For this review, take the finished solid that the model builds, in its own axes (mm). A direction names the side the tool comes from. Give positions to 0.01 mm unless a question says otherwise; leave off trailing zeros. Order: outer loops, then holes, each group sorted by start corner. A loop starts at its lowest first (then second) coordinate and runs counter-clockwise, first axis right, second up. Notation, with made-up numbers: (30, 84.25) -> (39, 84.25) arc R11 ccw to (39, 105.25) -> close; hole circle Ø4 at (-6.75, -16). An arc over 180 degrees is marked (long way). One line per item, written item: value. Start each with the question number.
from build123d import *

# Parameters (mm, degrees)
EXTRUDE_1_DEPTH          = 2
SKETCH_17_W              = 31.8
SKETCH_17_H              = 18
CUT_EXTRUDE_1_DEPTH      = 10
CHAMFER_1_SIZE           = 0.5
CHAMFER_3_SIZE           = 0.5
SKETCH_25_W              = 23.840125732
SKETCH_25_H              = 2
CUT_EXTRUDE_5_DEPTH      = 0.4
CUT_EXTRUDE_6_DEPTH      = 6
CUT_EXTRUDE_6_DEPTH_BACK = 6
SKETCH_28_R              = 0.9
EXTRUDE_3_DEPTH          = 1.2
CHAMFER_6_SIZE           = 0.4
SKETCH_29_R              = 1.6
CUT_EXTRUDE_7_DEPTH      = 3.2
SKETCH_30_R              = 3.5
CUT_EXTRUDE_8_DEPTH      = 10
CHAMFER_9_SIZE           = 0.4
FILLET_1_R               = 1
SKETCH_31_R              = 2.55
CUT_EXTRUDE_9_DEPTH      = 2
CHAMFER_10_SIZE          = 0.4
SKETCH_32_R              = 3.5
SKETCH_32_R_2            = 1.6
SKETCH_32_W              = 32.6
SKETCH_32_H              = 29.3
EXTRUDE_5_DEPTH          = 1.4


with BuildPart() as part:
    # Эскиз1 → Бобышка-Вытянуть1 (new body)
    with BuildSketch(Plane.XY):
        Polygon((42.994929839, 15.7), (0.265604814, 15.7), (-0.805070161, 15.7), (-0.805070161, -3.225667373), (-0.805070161, -27.24226554), (-0.805070161, -29), (41.213218599, -29), (42.994929839, -29), (42.994929839, 0), align=None)
    extrude(amount=EXTRUDE_1_DEPTH)

    # Эскиз17 → Вырез-Вытянуть1 (cut)
    with BuildSketch(Plane(origin=(0, 0, 0), x_dir=(-1, 0, 0), z_dir=(0, 0, -1))):
        with Locations((-21.094929839, 0)):
            Rectangle(SKETCH_17_W, SKETCH_17_H)
    extrude(amount=-CUT_EXTRUDE_1_DEPTH, mode=Mode.SUBTRACT)

    # Фаска1
    chamfer_1_edges = [part.edges().sort_by_distance(p)[0] for p in [
        (36.994929839, 0, 0),
        (21.094929839, -9, 0),
        (5.194929839, 0, 0),
        (21.094929839, 9, 0),
    ]]
    chamfer(chamfer_1_edges, length=CHAMFER_1_SIZE)

    # Фаска3
    chamfer_3_edges = [part.edges().sort_by_distance(p)[0] for p in [
        (21.094929839, 15.7, 0),
        (42.994929839, -6.65, 0),
        (21.094929839, -29, 0),
        (-0.805070161, -6.65, 0),
    ]]
    chamfer(chamfer_3_edges, length=CHAMFER_3_SIZE)

    # Эскиз25 → Вырез-Вытянуть5 (cut)
    with BuildSketch(Plane.XY.offset(2)):
        with Locations((22.524068439, -12.5)):
            Rectangle(SKETCH_25_W, SKETCH_25_H)
    extrude(amount=-CUT_EXTRUDE_5_DEPTH, mode=Mode.SUBTRACT)

    # Эскиз27 → Вырез-Вытянуть6 (cut, two sides: drawn at the far end of the back side and taken through both)
    with BuildSketch(Plane(origin=(0, 0.1, 0), x_dir=(-1, 0, 0), z_dir=(0, -1, 0)).offset(-CUT_EXTRUDE_6_DEPTH_BACK)):
        Polygon((-36.994929839, -2), (-36.994929839, -1.2), (-37.794929839, -2), align=None)
    extrude(amount=CUT_EXTRUDE_6_DEPTH + CUT_EXTRUDE_6_DEPTH_BACK, mode=Mode.SUBTRACT)

    # Эскиз28 → Бобышка-Вытянуть3 (add)
    with BuildSketch(Plane.XY.offset(2)):
        with Locations((7.894929839, 11.5)):
            Circle(SKETCH_28_R)
        with Locations((34.294929839, 11.5)):
            Circle(SKETCH_28_R)
        with Locations(Location((34.294929839, -11.5, 0), (0, 0, 180))):
            Circle(SKETCH_28_R)
        with Locations((7.894929839, -11.5)):
            Circle(SKETCH_28_R)
    extrude(amount=EXTRUDE_3_DEPTH)

    # Фаска6
    chamfer_6_edges = [part.edges().sort_by_distance(p)[0] for p in [
        (21.094929839, 9, 2),
        (21.094929839, -9, 2),
    ]]
    chamfer(chamfer_6_edges, length=CHAMFER_6_SIZE)

    # Эскиз29 → Вырез-Вытянуть7 (cut)
    with BuildSketch(Plane.XY.offset(2)):
        with Locations((2.594929839, 12.3)):
            Circle(SKETCH_29_R)
        with Locations((39.594929839, 12.3)):
            Circle(SKETCH_29_R)
        with Locations((39.594929839, -25.6)):
            Circle(SKETCH_29_R)
    extrude(amount=-CUT_EXTRUDE_7_DEPTH, mode=Mode.SUBTRACT)

    # Эскиз30 → Вырез-Вытянуть8 (cut)
    with BuildSketch(Plane.XY.offset(2)):
        with Locations((8.194929839, -21)):
            Circle(SKETCH_30_R)
    extrude(amount=-CUT_EXTRUDE_8_DEPTH, mode=Mode.SUBTRACT)

    # Фаска9
    chamfer_9_edges = [part.edges().sort_by_distance(p)[0] for p in [
        (4.694929839, -21, 0),
    ]]
    chamfer(chamfer_9_edges, length=CHAMFER_9_SIZE)

    # Скругление1
    # the kernel refuses this fillet: 1 mm, written as the material it takes off along each edge
    with BuildSketch(Plane(origin=(42.994929839, -29, -2), x_dir=(0, 1, 0), z_dir=(0, 0, 1)), Plane(origin=(42.994929839, 15.7, -2), x_dir=(-1, 0, 0), z_dir=(0, 0, 1))) as fillet_1_piece_1:
        with BuildLine():
            CenterArc((FILLET_1_R, FILLET_1_R), FILLET_1_R, 180, 90)
            Line((0, FILLET_1_R), (0, 0))
            Line((0, 0), (FILLET_1_R, 0))
        make_face()
    extrude(amount=6.5, mode=Mode.SUBTRACT)
    with BuildSketch(Plane(origin=(-0.805070161, -29, -2), x_dir=(0, 1, 0), z_dir=(0, 0, 1)), Plane(origin=(-0.805070161, 15.7, -2), x_dir=(1, 0, 0), z_dir=(0, 0, 1))) as fillet_1_piece_2:
        with BuildLine():
            CenterArc((FILLET_1_R, -FILLET_1_R), FILLET_1_R, 90, 90)
            Line((0, -FILLET_1_R), (0, 0))
            Line((0, 0), (FILLET_1_R, 0))
        make_face()
    extrude(amount=6.5, mode=Mode.SUBTRACT)
    with BuildSketch(Plane(origin=(0.528263172, 14.366666667, -0.833333333), x_dir=(0.816496580927726, 0.4082482904638629, 0.4082482904638631), z_dir=(-0.5773502691896258, 0.5773502691896258, 0.5773502691896258)), Plane(origin=(0.528263172, -27.666666667, -0.833333333), x_dir=(-0.4082482904638631, 0.8164965809277261, 0.4082482904638631), z_dir=(-0.5773502691896258, -0.5773502691896258, 0.5773502691896258))) as fillet_1_piece_3:
        with BuildLine():
            CenterArc((FILLET_1_R * 0.57735026919, -FILLET_1_R), FILLET_1_R, 90, 60)
            Line((-FILLET_1_R * 0.288675134595, -FILLET_1_R * 0.5), (0, 0))
            Line((0, 0), (FILLET_1_R * 0.57735026919, 0))
        make_face()
    extrude(amount=3.75277675, mode=Mode.SUBTRACT)
    with BuildSketch(Plane(origin=(41.661596505, 14.366666667, -0.833333333), x_dir=(-0.8164965809277261, 0.4082482904638622, 0.4082482904638635), z_dir=(0.5773502691896256, 0.577350269189626, 0.577350269189626)), Plane(origin=(41.661596505, -27.666666667, -0.833333333), x_dir=(0.4082482904638636, 0.8164965809277261, 0.40824829046386224), z_dir=(0.5773502691896261, -0.5773502691896256, 0.5773502691896256))) as fillet_1_piece_4:
        with BuildLine():
            CenterArc((FILLET_1_R * 0.57735026919, FILLET_1_R), FILLET_1_R, 210, 60)
            Line((-FILLET_1_R * 0.288675134595, FILLET_1_R * 0.5), (0, 0))
            Line((0, 0), (FILLET_1_R * 0.57735026919, 0))
        make_face()
    extrude(amount=3.75277675, mode=Mode.SUBTRACT)

    # Эскиз31 → Вырез-Вытянуть9 (cut)
    with BuildSketch(Plane(origin=(0, 0, 0), x_dir=(-1, 0, 0), z_dir=(0, 0, -1))):
        with Locations((-39.594929839, 12.3)):
            Circle(SKETCH_31_R)
        with Locations((-2.594929839, 12.3)):
            Circle(SKETCH_31_R)
        with Locations((-39.594929839, -25.6)):
            Circle(SKETCH_31_R)
    extrude(amount=-CUT_EXTRUDE_9_DEPTH, mode=Mode.SUBTRACT)

    # Фаска10
    # the kernel refuses this chamfer: 0.4 mm, written as the material it takes off along each edge
    with BuildSketch(Plane(origin=(39.594929839, -25.6, 0), x_dir=(-1, 0, 0), z_dir=(0, -1, 0))) as chamfer_10_piece_1:
        Polygon((2.55 + CHAMFER_10_SIZE, 0), (2.55, -CHAMFER_10_SIZE), (2.55, 0), align=None)
    revolve(axis=Axis((39.594929839, -25.6, 0), (0, 0, -1)), mode=Mode.SUBTRACT)
    with BuildSketch(Plane(origin=(2.594929839, 12.3, 0), x_dir=(-1, 0, 0), z_dir=(0, -1, 0))) as chamfer_10_piece_2:
        Polygon((2.55 + CHAMFER_10_SIZE, 0), (2.55, -CHAMFER_10_SIZE), (2.55, 0), align=None)
    revolve(axis=Axis((2.594929839, 12.3, 0), (0, 0, -1)), mode=Mode.SUBTRACT)
    with BuildSketch(Plane(origin=(39.594929839, 12.3, 0), x_dir=(-1, 0, 0), z_dir=(0, -1, 0))) as chamfer_10_piece_3:
        Polygon((2.55 + CHAMFER_10_SIZE, 0), (2.55, -CHAMFER_10_SIZE), (2.55, 0), align=None)
    revolve(axis=Axis((39.594929839, 12.3, 0), (0, 0, -1)), mode=Mode.SUBTRACT)

    # Эскиз32 → Бобышка-Вытянуть5 (add)
    with BuildSketch(Plane.XY.offset(2)):
        with BuildLine():
            Line((-0.805070161, 14.7), (-0.805070161, -28))
            ThreePointArc((-0.805070161, -28), (-0.512176942, -28.707106781), (0.194929839, -29))
            Line((0.194929839, -29), (41.994929839, -29))
            ThreePointArc((41.994929839, -29), (42.70203662, -28.707106781), (42.994929839, -28))
            Line((42.994929839, -28), (42.994929839, 14.7))
            ThreePointArc((42.994929839, 14.7), (42.70203662, 15.407106781), (41.994929839, 15.7))
            Line((41.994929839, 15.7), (0.194929839, 15.7))
            ThreePointArc((0.194929839, 15.7), (-0.512176942, 15.407106781), (-0.805070161, 14.7))
        make_face()
        with Locations((8.194929839, -21)):
            Circle(SKETCH_32_R, mode=Mode.SUBTRACT)
        with Locations((39.594929839, -25.6)):
            Circle(SKETCH_32_R_2, mode=Mode.SUBTRACT)
        with Locations((39.594929839, 12.3)):
            Circle(SKETCH_32_R_2, mode=Mode.SUBTRACT)
        with Locations((2.594929839, 12.3)):
            Circle(SKETCH_32_R_2, mode=Mode.SUBTRACT)
        with Locations((21.494929839, -0.35)):
            Rectangle(SKETCH_32_W, SKETCH_32_H, mode=Mode.SUBTRACT)
    extrude(amount=EXTRUDE_5_DEPTH)


solid = part.part
Q1. For line 1 along Y through (x, z) = (22, 0.7); line 2 along X through (y, z) = (-3.5, 0.6); line 3 along Y through (x, z) = (16.5, 2.5), list the stretches that pass through material, from the lowest coordinate up.
Q2. For pin 1 Ø5.5 at (x, y) = (8.19, -21) entering from +Z; pin 2 Ø1.4 at (x, y) = (8, -11.5) entering from +Z; pin 3 Ø4.5 at (x, y) = (14.5, -10.5) entering from +Z, all flat-tipped, find the tip position at first contact; note any pin that passes through.
Q3. Take a section at A-A (x = 19.5). State the section outline as (y, z) points.
Q4. Take a section at B-B (y = -21). State the section outline as (x, z) points.
Q5. Mouldability with a two-part tool opening along Y and no side actions: class faces 1 (the flat face through (0, 14, 0)), 2 (the cylindrical face through (7.232, 12.108, 2.592)), 3 (the cylindrical face through (-0.52, -28.7, 1.88)), 4 (the cylindrical face through (38.325, -26.574, 2.69)) as pulls with the +Y half, pulls with the -Y half, needs draft (parallel to the pull), parting line crosses it, or undercut.
Q6. Take a section at D-D (x = 7.5). State how many separate pieces and enclosed holes the cut face has, and give its area (3 significant figures).
Q7. Take a section at C-C (y = -25.6). State the section outline as (x, z) points (3 decimals), and give its area (3 significant figures).
Q8. For faces 5 (the flat face through (21, -15, 3)), 6 (the flat face through (21, 9, 1)), 7 (the flat face through (41.4, 12.3, 2)), list the 3-axis set-ups (+Z, -Z, +X, -X, +Y, -Y) from which the entire face can be reached by the end or side of a thin tool; tool diameter is ignored.
Answers below:
1. line 1: y = -29 to -9, 9 to 15.7
1. line 2: x = -0.81 to 5.19, 36.99 to 42.99
1. line 3: y = -29 to -15, 14.3 to 15.7
2. pin 1: passes through
2. pin 2: stops at z = 3.2
2. pin 3: stops at z = 2
3. outline: (-29, 0.5) -> (-28.5, 0) -> (-9.5, 0) -> (-9, 0.5) -> (-9, 1.6) -> (-9.4, 2) -> (-11.5, 2) -> (-11.5, 1.6) -> (-13.5, 1.6) -> (-13.5, 2) -> (-15, 2) -> (-15, 3.4) -> (-29, 3.4) -> close; (9, 0.5) -> (9.5, 0) -> (15.2, 0) -> (15.7, 0.5) -> (15.7, 3.4) -> (14.3, 3.4) -> (14.3, 2) -> (9.4, 2) -> (9, 1.6) -> close
4. outline: (-0.81, 0.5) -> (-0.31, 0) -> (4.29, 0) -> (4.69, 0.4) -> (4.69, 3.4) -> (-0.81, 3.4) -> close; (11.69, 0.4) -> (12.09, 0) -> (42.49, 0) -> (42.99, 0.5) -> (42.99, 3.4) -> (11.69, 3.4) -> close
5. face 1: needs draft
5. face 2: undercut
5. face 3: pulls with the -Y half
5. face 4: undercut
6. separate pieces: 3
6. enclosed holes: 0
6. area: 54.7 mm²
7. outline: (-0.805, 0.5) -> (-0.305, 0) -> (36.645, 0) -> (37.045, 0.4) -> (37.045, 2) -> (37.995, 2) -> (37.995, 3.4) -> (-0.805, 3.4) -> close; (41.195, 2) -> (42.145, 2) -> (42.145, 0.4) -> (42.52, 0.025) -> (42.995, 0.5) -> (42.995, 3.4) -> (41.195, 3.4) -> close
7. area: 134 mm²
8. face 5: +Z
8. face 6: +Z, -Z
8. face 7: -Z
